Design review of the part built by this model. Coordinates are the model's own, in mm. A direction names the side the tool comes from. Give positions to 0.01 mm unless a question says otherwise; leave off trailing zeros. Loops run counter-clockwise (first coordinate to the right, second up) from the corner with the lowest first, then second, coordinate; pieces in that order, holes last. Notation, with made-up numbers: (80, 30.5) -> (123, 30.5) arc R25 cw to (123, 65.5) -> close; hole circle Ø11 at (-36, 81). An arc over 180 degrees is marked (long way). Answer as CSV lines item,"result".
from build123d import *

# Parameters (mm, degrees)
SKETCH1_W           = 35
SKETCH1_H           = 35
SKETCH1_R           = 5.5
SKETCH1_R_2         = 2.5
SKETCH1_R_3         = 1.5
BOSS_EXTRUDE1_DEPTH = 10
FILLET1_R           = 3
SKETCH2_R           = 1.625
CUT_EXTRUDE1_DEPTH  = 10
SKETCH3_R           = 11.25
CUT_EXTRUDE2_DEPTH  = 3
SKETCH5_R           = 2.5
CUT_EXTRUDE4_DEPTH  = 3
FILLET2_R           = 2


with BuildPart() as part:
    # Sketch1 → Boss-Extrude1 (new body)
    with BuildSketch(Plane.XY):
        Rectangle(SKETCH1_W, SKETCH1_H)
        Circle(SKETCH1_R, mode=Mode.SUBTRACT)
        with Locations((-11.5, 11.5)):
            Circle(SKETCH1_R_2, mode=Mode.SUBTRACT)
        with Locations((11.5, 11.5)):
            Circle(SKETCH1_R_3, mode=Mode.SUBTRACT)
        with Locations((11.5, -11.5)):
            Circle(SKETCH1_R_2, mode=Mode.SUBTRACT)
        with Locations((-11.5, -11.5)):
            Circle(SKETCH1_R_3, mode=Mode.SUBTRACT)
    extrude(amount=BOSS_EXTRUDE1_DEPTH)

    # Fillet1
    fillet1_edges = [part.edges().sort_by_distance(p)[0] for p in [
        (17.5, -17.5, 5),
        (-17.5, -17.5, 5),
        (-17.5, 17.5, 5),
        (17.5, 17.5, 5),
    ]]
    fillet(fillet1_edges, radius=FILLET1_R)

    # Sketch2 → Cut-Extrude1 (cut)
    with BuildSketch(Plane.XY.offset(10)):
        with Locations((-8, 0)):
            Circle(SKETCH2_R)
        with Locations((0, 8)):
            Circle(SKETCH2_R)
        with Locations((8, 0)):
            Circle(SKETCH2_R)
        with Locations((0, -8)):
            Circle(SKETCH2_R)
    extrude(amount=-CUT_EXTRUDE1_DEPTH, mode=Mode.SUBTRACT)

    # Sketch3 → Cut-Extrude2 (cut)
    with BuildSketch(Plane.XY.offset(10)):
        Circle(SKETCH3_R)
    extrude(amount=-CUT_EXTRUDE2_DEPTH, mode=Mode.SUBTRACT)

    # Sketch5 → Cut-Extrude4 (cut)
    # profile 1 of 2: a face of its own
    with BuildSketch(Plane(origin=(0, 0, 0), x_dir=(-1, 0, 0), z_dir=(0, 0, -1))):
        with BuildLine():
            Line((-15.742640687, -7.257359313), (-17.5, -9.014718626))
            Line((-17.5, -9.014718626), (-17.5, -14.5))
            ThreePointArc((-17.5, -14.5), (-16.621320344, -16.621320344), (-14.5, -17.5))
            Line((-14.5, -17.5), (-9.014718626, -17.5))
            Line((-9.014718626, -17.5), (-7.257359313, -15.742640687))
            ThreePointArc((-7.257359313, -15.742640687), (-7.257359313, -7.257359313), (-15.742640687, -7.257359313))
        make_face()
        with Locations((-11.5, -11.5)):
            Circle(SKETCH5_R, mode=Mode.SUBTRACT)
    # profile 2 of 2: a face of its own
    with BuildSketch(Plane(origin=(0, 0, 0), x_dir=(-1, 0, 0), z_dir=(0, 0, -1))):
        with BuildLine():
            Line((9.014718626, 17.5), (7.257359313, 15.742640687))
            ThreePointArc((7.257359313, 15.742640687), (7.257359313, 7.257359313), (15.742640687, 7.257359313))
            Line((15.742640687, 7.257359313), (17.5, 9.014718626))
            Line((17.5, 9.014718626), (17.5, 14.5))
            ThreePointArc((17.5, 14.5), (16.621320344, 16.621320344), (14.5, 17.5))
            Line((14.5, 17.5), (9.014718626, 17.5))
        make_face()
        with Locations((11.5, 11.5)):
            Circle(SKETCH5_R, mode=Mode.SUBTRACT)
    extrude(amount=-CUT_EXTRUDE4_DEPTH, mode=Mode.SUBTRACT)

    # Fillet2
    # the kernel refuses this fillet: 2 mm, written as the material it takes off along each edge
    with BuildSketch(Plane(origin=(-9.014718626, 17.5, -11.10730464), x_dir=(0.6704488170211711, -0.7419557828839344, 0), z_dir=(0, 0, 1))) as fillet2_piece_1:
        with BuildLine():
            CenterArc((4.462663268, 1.95555393), FILLET2_R, 137.89828583, 120)
            Line((2.978751702, 3.296451564), (2.830360546, 3.430541327))
            Line((2.830360546, 3.430541327), (-0.148391157, 0.134089763))
            Line((-0.148391157, 0.134089763), (0.010112612, -0.199744174))
            ThreePointArc((0.010112612, -0.199744174), (2.492214989, -0.074080742), (4.001438073, -0.195555393))
            Line((4.001438073, -0.195555393), (4.043367636, 0))
        make_face()
    extrude(amount=14.10730464, mode=Mode.SUBTRACT)
    with BuildSketch(Plane(origin=(-17.5, 9.014718626, -11.10730464), x_dir=(0, -1, 0), z_dir=(0, 0, 1)), Plane(origin=(17.5, -9.014718626, -11.10730464), x_dir=(0, 1, 0), z_dir=(0, 0, 1))) as fillet2_piece_2:
        with BuildLine():
            CenterArc((4.442921856, 2), FILLET2_R, 150, 120)
            Line((2.710871048, 3), (2.537665968, 3.1))
            ThreePointArc((2.537665968, 3.1), (1.615937957, 1.898780669), (-0.141421356, 0.141421356))
            Line((-0.141421356, 0.141421356), (0, -0.2))
            Line((0, -0.2), (4.442921856, -0.2))
            Line((4.442921856, -0.2), (4.442921856, 0))
        make_face()
    extrude(amount=14.10730464, mode=Mode.SUBTRACT)
    with BuildSketch(Plane(origin=(9.014718626, -17.5, -11.10730464), x_dir=(-1, 0, 0), z_dir=(0, 0, 1))) as fillet2_piece_3:
        with BuildLine():
            CenterArc((4.442921856, -2), FILLET2_R, 90, 120)
            Line((2.710871048, -3), (2.537665968, -3.1))
            ThreePointArc((2.537665968, -3.1), (1.615937957, -1.898780669), (-0.141421356, -0.141421356))
            Line((-0.141421356, -0.141421356), (0, 0.2))
            Line((0, 0.2), (4.442921856, 0.2))
            Line((4.442921856, 0.2), (4.442921856, 0))
        make_face()
    extrude(amount=14.10730464, mode=Mode.SUBTRACT)


solid = part.part
Q1. The part is to be moulded in two halves that separate along X. For faces 1 (the flat face through (0, 17.5, 5)), 2 (the flat face through (17.5, 0, 5)), 3 (the cylindrical face through (-1.19, -5.37, 3.45)), say which applies: pulls with the +X half, pulls with the -X half, needs draft (parallel to the pull), parting line crosses it, or undercut.
Filled sheet:
face 1,"needs draft"
face 2,"pulls with the +X half"
face 3,"undercut"
Q2. We need section D-D, the plane x = 1. State the section outline as (y, z) points, and give its area (3 significant figures).
Filled sheet:
outline,"(-17.5, 0) -> (-9.28, 0) -> (-9.28, 7) -> (-11.21, 7) -> (-11.21, 10) -> (-17.5, 10) -> close; (-6.72, 0) -> (-5.41, 0) -> (-5.41, 7) -> (-6.72, 7) -> close; (5.41, 0) -> (6.72, 0) -> (6.72, 7) -> (5.41, 7) -> close; (9.28, 0) -> (17.5, 0) -> (17.5, 10) -> (11.21, 10) -> (11.21, 7) -> (9.28, 7) -> close"
area,"171 mm^2"
Q3. We need section C-C, the plane y = 8. State the section outline as (x, z) points (3 decimals), and give its area (3 significant figures).
Filled sheet:
outline,"(-17.5, 3) -> (-6.627, 3) -> (-6.627, 0) -> (-1.625, 0) -> (-1.625, 7) -> (-7.91, 7) -> (-7.91, 10) -> (-17.5, 10) -> close; (1.625, 0) -> (17.5, 0) -> (17.5, 10) -> (7.91, 10) -> (7.91, 7) -> (1.625, 7) -> close"
area,"247 mm^2"
Q4. We need section A-A, the plane y = 0. State the section outline as (x, z) points (3 decimals).
Filled sheet:
outline,"(-17.5, 0) -> (-9.625, 0) -> (-9.625, 7) -> (-11.25, 7) -> (-11.25, 10) -> (-17.5, 10) -> close; (-6.375, 0) -> (-5.5, 0) -> (-5.5, 7) -> (-6.375, 7) -> close; (5.5, 0) -> (6.375, 0) -> (6.375, 7) -> (5.5, 7) -> close; (9.625, 0) -> (17.5, 0) -> (17.5, 10) -> (11.25, 10) -> (11.25, 7) -> (9.625, 7) -> close"
Q5. Clearance check with flat-ended pins moving along their axes: pin 1 Ø17.5 at (x, y) = (0, 0) entering from +Z; pin 2 Ø3 at (x, y) = (-8, 0) entering from -Z; pin 3 Ø14 at (x, y) = (-9, 13) entering from -Z; pin 4 Ø8 at (x, y) = (11.5, -11.5) entering from -Z. State where each tip first meets the part, or that it passes through.
Filled sheet:
pin 1,"stops at z = 7"
pin 2,"passes through"
pin 3,"stops at z = 0"
pin 4,"stops at z = 3"
Q6. For faces 4 (the cylindrical face through (-7.18, 7.336, 1.479)), 5 (the cylindrical face through (6.289, -16.525, 1.479)), 6 (the flat face through (5, 3, 7)), list the 3-axis set-ups (+Z, -Z, +X, -X, +Y, -Y) from which the entire face can be reached by the end or side of a thin tool; tool diameter is ignored.
Filled sheet:
face 4,"-Z"
face 5,"-Z, +X"
face 6,"+Z"
Q7. We need section B-B, the plane z = 5.5. State how many separate pieces and enclosed holes the cut face has, and give its area (3 significant figures).
Filled sheet:
separate pieces,"1"
enclosed holes,"9"
area,"1,040 mm^2"
Q8. To check wall thickness, follow probe 1 along Y at (x, z) = (-11.5, 3.5); probe 2 along Y at (x, z) = (0, 3.25) (3 decimals); probe 3 along Y at (x, z) = (-13.5, 8.25). State the ranges of each line that lie inside material, in increasing order. Write a range as from..to.
Filled sheet:
probe 1,"y = -17.5..-13, -10..9, 14..17.5"
probe 2,"y = -17.5..-9.625, -6.375..-5.5, 5.5..6.375, 9.625..17.5"
probe 3,"y = -17.5..10, 13..17.5"
